from build123d import *

# Parameters (mm, degrees)
SKETCH_2_R      = 1.6
SKETCH_2_R_2    = 2.6
SKETCH_2_R_3    = 11.1
SKETCH_2_R_4    = 3.655
EXTRUDE_1_DEPTH = 6
FILLET_1_R      = 0.3
CHAMFER_1_SIZE  = 1


with BuildPart() as part:
    # Эскиз2 → Бобышка-Вытянуть1 (new body)
    with BuildSketch(Plane(origin=(0, 0, 0), x_dir=(0, 0, -1), z_dir=(1, 0, 0))):
        with BuildLine():
            Line((-30, 47.1129), (30, 47.1129))
            ThreePointArc((30, 47.1129), (37.071067812, 44.183967812), (40, 37.1129))
            Line((40, 37.1129), (40, -30.391408151))
            ThreePointArc((40, -30.391408151), (39.238795325, -34.218242474), (37.071067812, -37.462475962))
            Line((37.071067812, -37.462475962), (2.828427125, -71.70511665))
            ThreePointArc((2.828427125, -71.70511665), (0, -72.876689525), (-2.828427125, -71.70511665))
            Line((-2.828427125, -71.70511665), (-37.071067812, -37.462475962))
            ThreePointArc((-37.071067812, -37.462475962), (-39.238795325, -34.218242474), (-40, -30.391408151))
            Line((-40, -30.391408151), (-40, 37.1129))
            ThreePointArc((-40, 37.1129), (-37.071067812, 44.183967812), (-30, 47.1129))
        make_face()
        with Locations((-21.913410217, -46.3871)):
            Circle(SKETCH_2_R, mode=Mode.SUBTRACT)
        with Locations((17.25, -19.8871)):
            Circle(SKETCH_2_R_2, mode=Mode.SUBTRACT)
        with Locations((-17.25, -19.8871)):
            Circle(SKETCH_2_R_2, mode=Mode.SUBTRACT)
        with Locations((0.0069, -46.3871)):
            Circle(SKETCH_2_R_3, mode=Mode.SUBTRACT)
        with Locations((-25, 37.1129)):
            Circle(SKETCH_2_R_4, mode=Mode.SUBTRACT)
        with Locations((25, 37.1129)):
            Circle(SKETCH_2_R_4, mode=Mode.SUBTRACT)
        with Locations((0.0069, -24.466789783)):
            Circle(SKETCH_2_R, mode=Mode.SUBTRACT)
        with Locations((21.927210217, -46.3871)):
            Circle(SKETCH_2_R, mode=Mode.SUBTRACT)
        with Locations((0.0069, -68.307410217)):
            Circle(SKETCH_2_R, mode=Mode.SUBTRACT)
    extrude(amount=EXTRUDE_1_DEPTH)

    # Скругление1
    fillet_1_edges = [part.edges().sort_by_distance(p)[0] for p in [
        (6, 44.183967812, 37.071067812),
        (6, 3.360745925, 40),
        (6, -34.218242474, 39.238795325),
        (6, -54.583796306, 19.949747468),
        (6, -72.876689525, 0),
        (6, -54.583796306, -19.949747468),
        (6, -34.218242474, -39.238795325),
        (6, 3.360745925, -40),
        (6, 44.183967812, -37.071067812),
        (6, -46.3871, 11.0931),
        (6, 47.1129, 0),
    ]]
    fillet(fillet_1_edges, radius=FILLET_1_R)

    # Фаска1
    chamfer_1_edges = [part.edges().sort_by_distance(p)[0] for p in [
        (6, -24.466789783, 1.5931),
        (6, -46.3871, 23.513410217),
        (6, -46.3871, -20.327210217),
        (6, -68.307410217, 1.5931),
        (6, -19.8871, -14.65),
        (6, -19.8871, 19.85),
    ]]
    chamfer(chamfer_1_edges, length=CHAMFER_1_SIZE)


solid = part.part
Verification items for the finished model (mm, model axes). Coordinates: 2 decimals unless noted, no trailing zeros.
1. Scan lines: line 1 (Z direction, x = 4, y = 34.5); line 2 (Z direction, x = 5.75, y = -21); line 3 (Z direction, x = 5.75, y = -30.5). Record each from-to range of solid material in increasing order.
Results found:
line 1: z = -40 to -27.56, -22.44 to 22.44, 27.56 to 40
line 2: z = -40 to -20.41, -14.09 to 14.09, 20.41 to 40
line 3: z = -40 to 40
2. Go/stop test with flat-tipped pins: pin 1 Ø5 at (y, z) = (-24.47, -0.01) entering from +X; pin 2 Ø6.5 at (y, z) = (37.11, -25) entering from +X; pin 3 Ø4 at (y, z) = (-46.39, -21.93) entering from +X. Record where each tip stops, or that it passes through.
Results found:
pin 1: stops at x = 5.9
pin 2: passes through
pin 3: stops at x = 5.4
3. Sectioned sample at A-A, the plane x = 1. Give the number of separate pieces and of enclosed holes in the cut face, and give its area (3 significant figures).
Results found:
separate pieces: 1
enclosed holes: 9
area: 7,540 mm2
4. Release check for a two-part mould opening along Y. For faces 1 (the face through (2.46, -26.03, 0.34)), 2 (the face through (2.81, 44.261, -36.993)), 3 (the face through (3, 4, -40)), 4 (the face through (2.81, -34.269, 39.218)) record: +Y half, -Y half, draft (parallel to the pull), parting line (faces both ways), or undercut.
Results found:
face 1: undercut
face 2: +Y half
face 3: draft
face 4: -Y half
